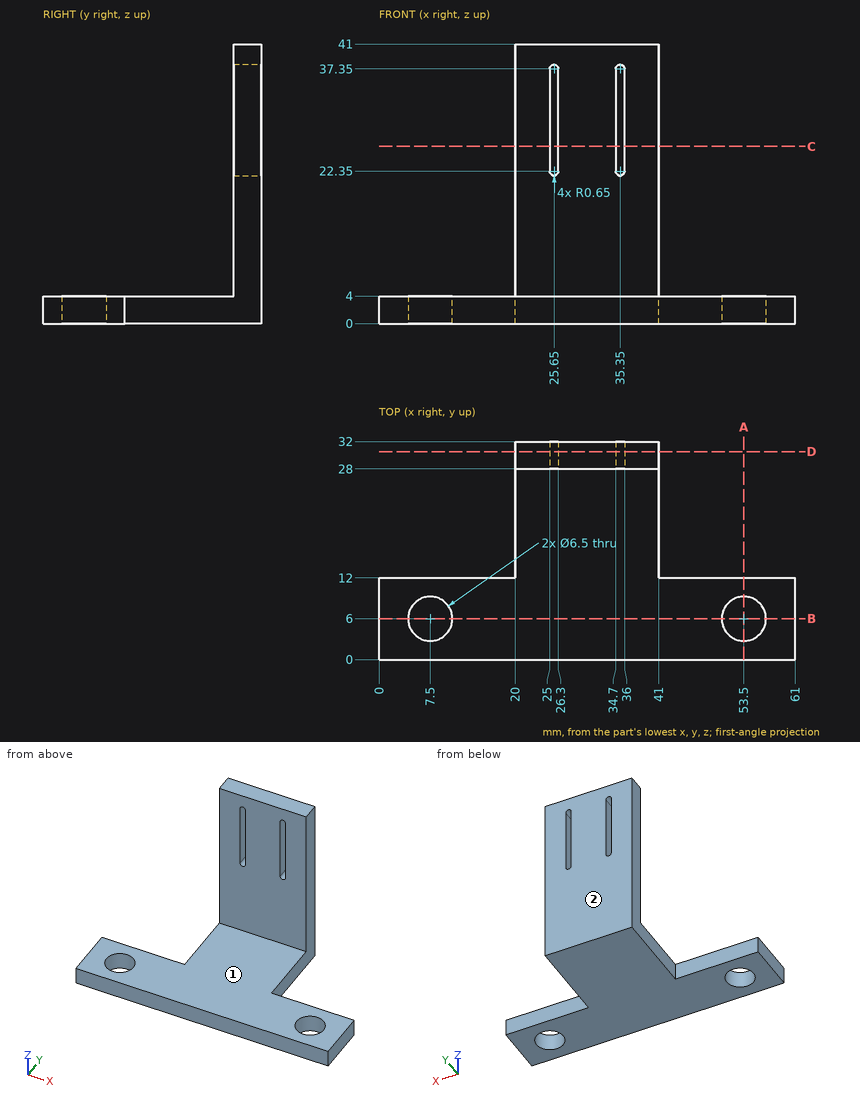
The figure shows three views and two pictorial views of one solid part (mm, origin at its lowest corner). Answer the questions. A direction names the side the tool comes from. Give positions to 0.01 mm unless a question says otherwise; leave off trailing zeros. Loops run counter-clockwise (first coordinate to the right, second up) from the corner with the lowest first, then second, coordinate; pieces in that order, holes last. Notation, with made-up numbers: (-22.5, 79.5) - (31.5, 79.5) arc R7 cw to (31.5, 85.5) - close; hole circle Ø4 at (-39, 57.5). An arc over 180 degrees is marked (long way). Answer in a Markdown table with one row per item.
(1) Section B-B (y = 6) is taken. Give the vertices of the cut face in (x, z), and give its area (3 significant figures).
Results list:
| item | result |
|---|---|
| outline | (0, 0) - (4.25, 0) - (4.25, 4) - (0, 4) - close; (10.75, 0) - (50.25, 0) - (50.25, 4) - (10.75, 4) - close; (56.75, 0) - (61, 0) - (61, 4) - (56.75, 4) - close |
| area | 192 mm² |
(2) Section A-A (x = 53.5) is taken. Give the vertices of the cut face in (y, z).
Results list:
| item | result |
|---|---|
| outline | (0, 0) - (2.75, 0) - (2.75, 4) - (0, 4) - close; (9.25, 0) - (12, 0) - (12, 4) - (9.25, 4) - close |
(3) Section C-C (z = 26) is taken. Give the vertices of the cut face in (x, y), and give its area (3 significant figures).
Results list:
| item | result |
|---|---|
| outline | (20, 28) - (25, 28) - (25, 32) - (20, 32) - close; (26.3, 28) - (34.7, 28) - (34.7, 32) - (26.3, 32) - close; (36, 28) - (41, 28) - (41, 32) - (36, 32) - close |
| area | 73.6 mm² |
(4) Consider L1, parallel to Y at x = 53.5, z = 1.4; L2, parallel to Z at x = 36, y = 22.5; L3, parallel to Y at x = 21.5, z = 19.5. Determine where each line is inside the solid, lowest interval first. Write a range as [from, to].
Results list:
| item | result |
|---|---|
| L1 | y = [0, 2.75], [9.25, 12] |
| L2 | z = [0, 4] |
| L3 | y = [28, 32] |
(5) Flat-ended cylindrical pins translate along their axes: pin 1 Ø3 at (y, z) = (30, 32) entering from -X; pin 2 Ø4.5 at (y, z) = (30, 31) entering from +X; pin 3 Ø23 at (x, z) = (26, 22) entering from -Y. Find the tip coordinate at first contact, or state that the pin passes through.
Results list:
| item | result |
|---|---|
| pin 1 | stops at x = 20 |
| pin 2 | stops at x = 41 |
| pin 3 | stops at y = 28 |
(6) Section D-D (y = 30.5) is taken. Give the vertices of the cut face in (x, z).
Results list:
| item | result |
|---|---|
| outline | (20, 0) - (41, 0) - (41, 41) - (20, 41) - close; hole (25, 22.35) arc R0.65 ccw to (26.3, 22.35) - (26.3, 37.35) arc R0.65 ccw to (25, 37.35) - close; hole (34.7, 22.35) arc R0.65 ccw to (36, 22.35) - (36, 37.35) arc R0.65 ccw to (34.7, 37.35) - close |
(7) A tool of negligible diameter and unlimited length cuts with its end or side. For the marked faces 1 and 2, from which of +Z, -Z, +X, -X, +Y, -Y can it reach the whole face along a straight path? Write none if from no direction.
Results list:
| item | result |
|---|---|
| face 1 | +Z, +X, -X, -Y |
| face 2 | +Z, -Z, +X, -X, +Y |
